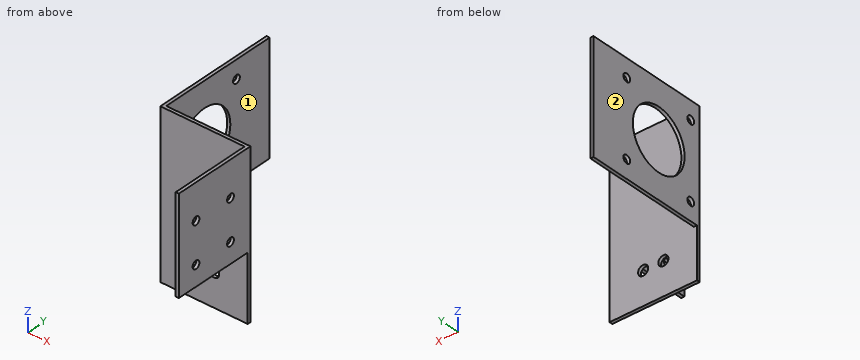
```python
from build123d import *

# Parameters (mm, degrees)
SKETCH1_W           = 69.85
SKETCH1_H           = 50.8
BOSS_EXTRUDE1_DEPTH = 2
SKETCH2_W           = 54.8
SKETCH2_H           = 69.85
BOSS_EXTRUDE2_DEPTH = 2
SKETCH3_W           = 2
SKETCH3_H           = 69.85
BOSS_EXTRUDE3_DEPTH = 76.2
SKETCH4_R           = 19.05
SKETCH4_R_2         = 2.5
CUT_EXTRUDE1_DEPTH  = 122.410689912
SKETCH5_R           = 2.5
SKETCH5_W           = 9.525
SKETCH5_H           = 52.8
CUT_EXTRUDE2_DEPTH  = 76.2
SKETCH6_W           = 54.8
SKETCH6_H           = 2
BOSS_EXTRUDE4_DEPTH = 41.275
SKETCH7_R           = 3.175
CUT_EXTRUDE3_DEPTH  = 116.130515612


with BuildPart() as part:
    # Sketch1 → Boss-Extrude1 (new body)
    with BuildSketch(Plane(origin=(0, 0, 0), x_dir=(0, 0, -1), z_dir=(1, 0, 0))):
        Rectangle(SKETCH1_W, SKETCH1_H)
    extrude(amount=-BOSS_EXTRUDE1_DEPTH)

    # Sketch2 → Boss-Extrude2 (add)
    with BuildSketch(Plane(origin=(0, 25.4, 0), x_dir=(1, 0, 0), z_dir=(0, 1, 0))):
        with Locations((-27.4, 0)):
            Rectangle(SKETCH2_W, SKETCH2_H)
    extrude(amount=BOSS_EXTRUDE2_DEPTH)

    # Sketch3 → Boss-Extrude3 (add)
    with BuildSketch(Plane(origin=(0, 27.4, 0), x_dir=(1, 0, 0), z_dir=(0, 1, 0))):
        with Locations((-53.8, 0)):
            Rectangle(SKETCH3_W, SKETCH3_H)
    extrude(amount=BOSS_EXTRUDE3_DEPTH)

    # Sketch4 → Cut-Extrude1 (cut, through all)
    with BuildSketch(Plane(origin=(-52.8, 0, 0), x_dir=(0, 0, -1), z_dir=(1, 0, 0))):
        with Locations((0, 55.567958179)):
            Circle(SKETCH4_R)
        with Locations((23.55, 79.117958179)):
            Circle(SKETCH4_R_2)
        with Locations((-23.55, 79.117958179)):
            Circle(SKETCH4_R_2)
        with Locations((-23.55, 32.017958179)):
            Circle(SKETCH4_R_2)
        with Locations((23.55, 32.017958179)):
            Circle(SKETCH4_R_2)
    extrude(amount=-CUT_EXTRUDE1_DEPTH, mode=Mode.SUBTRACT)

    # Sketch5 → Cut-Extrude2 (cut)
    with BuildSketch(Plane(origin=(0, 0, 0), x_dir=(0, 0, -1), z_dir=(1, 0, 0))):
        with Locations((-12.7, 12.7)):
            Circle(SKETCH5_R)
        with Locations((12.7, 12.7)):
            Circle(SKETCH5_R)
        with Locations((12.7, -12.7)):
            Circle(SKETCH5_R)
        with Locations((-12.7, -12.7)):
            Circle(SKETCH5_R)
        with Locations((30.1625, 1)):
            Rectangle(SKETCH5_W, SKETCH5_H)
    extrude(amount=-CUT_EXTRUDE2_DEPTH, mode=Mode.SUBTRACT)

    # Sketch6 → Boss-Extrude4 (add)
    with BuildSketch(Plane(origin=(0, 0, -25.4), x_dir=(-1, 0, 0), z_dir=(0, 0, -1))):
        with Locations((27.4, 26.4)):
            Rectangle(SKETCH6_W, SKETCH6_H)
    extrude(amount=BOSS_EXTRUDE4_DEPTH)

    # Sketch7 → Cut-Extrude3 (cut, through all)
    with BuildSketch(Plane(origin=(0, 27.4, 0), x_dir=(1, 0, 0), z_dir=(0, 1, 0))):
        with Locations(Location((-33.75, 46.0375, 0), (0, 0, 270))):
            Circle(SKETCH7_R)
        with Locations(Location((-21.05, 46.0375, 0), (0, 0, 270))):
            Circle(SKETCH7_R)
    extrude(amount=-CUT_EXTRUDE3_DEPTH, mode=Mode.SUBTRACT)


solid = part.part
```
Verification items for the finished model (mm, model axes). Face numbers are marked on the shaded views. A direction names the side the tool comes from. Coordinates: 2 decimals unless noted, no trailing zeros. Order: outer loops, then holes, each group sorted by start corner. A loop starts at its lowest first (then second) coordinate and runs counter-clockwise, first axis right, second up. Notation, with made-up numbers: (-25, 12.5) - (-17, 12.5) arc R19 cw to (-17, 34.5) - close; hole circle Ø9 at (40, 6). An arc over 180 degrees is marked (long way). Return JSON: item names as keys, results as strings.
(1) Go/stop test with flat-tipped pins: pin 1 (1.6 mm diameter, centred on x = -1.5, y = -3, fed in from -Z); pin 2 (4 mm diameter, centred on x = -39.5, z = -31, fed in from +Y); pin 3 (6.5 mm diameter, centred on y = 79.12, z = -23.55, fed in from +X). Record where each tip stops, or that it passes through.
Filled sheet:
{"pin 1": "stops at z = -25.4", "pin 2": "stops at y = 27.4", "pin 3": "stops at x = -52.8"}
(2) Section check A-A, the plane x = -21.05. Record the cut outline in (y, z) (1 decimal), and give its area (4 significant figures).
Filled sheet:
{"outline": "(25.4, -66.7) - (27.4, -66.7) - (27.4, -49.2) - (25.4, -49.2) - close; (25.4, -42.9) - (27.4, -42.9) - (27.4, 34.9) - (25.4, 34.9) - close", "area": "190.5 mm^2"}
(3) Section check D-D, the plane z = 0. Record the cut outline in (x, y).
Filled sheet:
{"outline": "(-54.8, 25.4) - (-2, 25.4) - (-2, -25.4) - (0, -25.4) - (0, 27.4) - (-52.8, 27.4) - (-52.8, 36.52) - (-54.8, 36.52) - close; (-54.8, 74.62) - (-52.8, 74.62) - (-52.8, 103.6) - (-54.8, 103.6) - close"}
(4) Section check C-C, the plane y = 12.7. Record the cut outline in (x, z) (3 decimals).
Filled sheet:
{"outline": "(-2, -25.4) - (0, -25.4) - (0, -15.2) - (-2, -15.2) - close; (-2, -10.2) - (0, -10.2) - (0, 10.2) - (-2, 10.2) - close; (-2, 15.2) - (0, 15.2) - (0, 34.925) - (-2, 34.925) - close"}
(5) Thickness scan on line 1 along Y through (x, z) = (-54, 23); line 2 along X through (y, z) = (70, -32.5); line 3 along Y through (x, z) = (-20, -18). Record the ranges inside material, lowest first.
Filled sheet:
{"line 1": "y = 25.4 to 29.58, 34.46 to 76.68, 81.56 to 103.6", "line 2": "x = -54.8 to -52.8", "line 3": "y = 25.4 to 27.4"}
(6) Access from +Z, -Z, +X, -X, +Y, -Y to the whole of each face (thin tool, end or side, straight path). Record for the marked faces 1 and 2.
Filled sheet:
{"face 1": "+Z, -Z, +X, +Y", "face 2": "+Z, -Z, -X, +Y, -Y"}
(7) Section check B-B, the plane z = 12.7. Record the cut outline in (x, y).
Filled sheet:
{"outline": "(-54.8, 25.4) - (-2, 25.4) - (-2, 15.2) - (0, 15.2) - (0, 27.4) - (-52.8, 27.4) - (-52.8, 41.37) - (-54.8, 41.37) - close; (-54.8, 69.77) - (-52.8, 69.77) - (-52.8, 103.6) - (-54.8, 103.6) - close; (-2, -25.4) - (0, -25.4) - (0, -15.2) - (-2, -15.2) - close; (-2, -10.2) - (0, -10.2) - (0, 10.2) - (-2, 10.2) - close"}
